```python
from build123d import *

# Parameters (mm, degrees)
F0_W      = 103.65
F0_H      = 64
F0_R      = 1.5
F1_DEPTH  = 1.5
F2_W      = 9
F2_H      = 11
F3_DEPTH  = 16
F4_W      = 7
F4_H      = 7
F4_H_2    = 4
F5_DEPTH  = 1.5
F6_R      = 3.25
F7_DEPTH  = 6
F8_W      = 7
F8_H      = 4.0027049468
F8_H_2    = 1.5
F8_H_3    = 1.4972950532
F9_DEPTH  = 1.5
F10_R     = 3.25
F11_DEPTH = 8
F12_SIZE  = 0.5
F13_SIZE  = 0.5


with BuildPart() as f1:
    # F0 (on Top) → F1 (new body)
    with BuildSketch(Plane.XY):
        Rectangle(F0_W, F0_H)
        with Locations((-48.825, -29)):
            Circle(F0_R, mode=Mode.SUBTRACT)
        with Locations((48.825, -29)):
            Circle(F0_R, mode=Mode.SUBTRACT)
        with Locations((-48.825, 29)):
            Circle(F0_R, mode=Mode.SUBTRACT)
        with Locations((48.825, 29)):
            Circle(F0_R, mode=Mode.SUBTRACT)
    extrude(amount=F1_DEPTH)

    # F2 (on face) → F3 (join)
    with BuildSketch(Plane.YZ.offset(51.825)):
        with Locations((-9.7, 7)):
            Rectangle(F2_W, F2_H)
    extrude(amount=-F3_DEPTH)

    # F4 (on face) → F5 (join)
    with BuildSketch(Plane.YZ.offset(51.825)):
        with Locations((5.9, 2)):
            Rectangle(F4_W, F4_H)
        with Locations((5.9, 3.5)):
            Rectangle(F4_W, F4_H_2)
    extrude(amount=F5_DEPTH)

    # F6 (on face) → F7 (join)
    with BuildSketch(Plane.YZ.offset(53.325)):
        with Locations((5.9, 2)):
            Circle(F6_R)
    extrude(amount=F7_DEPTH)

    # F8 (on face) → F9 (join)
    with BuildSketch(Plane(origin=(-51.825, 0, 0), x_dir=(0, -1, 0), z_dir=(-1, 0, 0))):
        with Locations((-3, 3.5013524734)):
            Rectangle(F8_W, F8_H)
        with Locations((-3, 0.75)):
            Rectangle(F8_W, F8_H_2)
        with Locations((-3, -0.7486475266)):
            Rectangle(F8_W, F8_H_3)
    extrude(amount=F9_DEPTH)

    # F10 (on face) → F11 (join)
    with BuildSketch(Plane(origin=(-53.325, 0, 0), x_dir=(0, -1, 0), z_dir=(-1, 0, 0))):
        with Locations((-3, 2.0027049468)):
            Circle(F10_R)
    extrude(amount=F11_DEPTH)

    # F12
    f12_edges = [f1.edges().sort_by_distance(p)[0] for p in [
        (-61.325, 6.25, 2.002705),
    ]]
    chamfer(f12_edges, length=F12_SIZE)

    # F13
    f13_edges = [f1.edges().sort_by_distance(p)[0] for p in [
        (59.325, 2.65, 2),
    ]]
    chamfer(f13_edges, length=F13_SIZE)


solid = f1.part
```
Can you work these out from the model? Positions are in its coordinate system, mm. A direction names the side the tool comes from. Give positions to 0.01 mm unless a question says otherwise; leave off trailing zeros. Order: outer loops, then holes, each group sorted by start corner. A loop starts at its lowest first (then second) coordinate and runs counter-clockwise, first axis right, second up. Notation, with made-up numbers: (33, -7) - (53, -7) arc R16 cw to (53, 22) - close; hole circle Ø4 at (-27.5, 64). An arc over 180 degrees is marked (long way). Use a Markdown table: item, result. Add a question column.
Q1. Please list where these lines run through material, in increasing order: line 1 along X through (y, z) = (5, 2.75) (3 decimals); line 2 along Z through (x, y) = (25, 24); line 3 along X through (y, z) = (-5.5, 11.25) (3 decimals).
Q2. On a 3-axis mill with a long thin cutter (end or side, diameter ignored), from which of +Z, -Z, +X, -X, +Y, -Y can I reach the whole of each face in a straight line? I mean faces 1 (the cylindrical face through (56.037, 3.321, 0.022)), 2 (the flat face through (44, -5.2, 7)), 3 (the flat face through (51.825, 6, 4)). Say none if no direction works.
Q3. If we section it at A-A on y = -29: Write out the boundary of the cut face in (x, z) (3 decimals).
Q4. I'm going to push flat-ended pins straight in: pin 1 (1.2 mm diameter, centred on x = -52.5, z = 0.5, fed in from -Y); pin 2 (5 mm diameter, centred on x = 48.825, y = 29, fed in from +Z); pin 3 (8 mm diameter, centred on x = 39, y = 12, fed in from -Z). Where does each tip first touch, or does it pass through?
Q5. If we section it at C-C on y = -11.5: Write out the boundary of the cut face in (x, z) (3 decimals), plus the area to 3 significant figures.
Q6. If we section it at D-D on z = 9.5: Write out the boundary of the cut face in (x, y) (3 decimals), plus the area to 3 significant figures.
Q7. If we section it at B-B on x = -49: Write out the boundary of the cut face in (y, z), plus the area to 3 significant figures.
Q8. If we mould it in two halves opening along X, with no side actions, what happens to faces 4 (the flat face through (51.825, -11, 5)), 5 (the cylindrical face through (48.63, -27.513, 0.74)), 6 (the flat face through (-61.325, 3, 2))? For each: released by +X, released by -X, zero draft, split by the parting line, or undercut.
Answers follow:
| question | item | result |
|---|---|---|
| 1 | line 1 | x = -61.325 to -51.825, 51.825 to 59.325 |
| 1 | line 2 | z = 0 to 1.5 |
| 1 | line 3 | x = 35.825 to 51.825 |
| 2 | face 1 | +X |
| 2 | face 2 | +Z, +X, -X, +Y |
| 2 | face 3 | +Z, +Y |
| 3 | outline | (-51.825, 0) - (-50.325, 0) - (-50.325, 1.5) - (-51.825, 1.5) - close; (-47.325, 0) - (47.325, 0) - (47.325, 1.5) - (-47.325, 1.5) - close; (50.325, 0) - (51.825, 0) - (51.825, 1.5) - (50.325, 1.5) - close |
| 4 | pin 1 | stops at y = -0.5 |
| 4 | pin 2 | stops at z = 1.5 |
| 4 | pin 3 | stops at z = 0 |
| 5 | outline | (-51.825, 0) - (51.825, 0) - (51.825, 12.5) - (35.825, 12.5) - (35.825, 1.5) - (-51.825, 1.5) - close |
| 5 | area | 331 mm^2 |
| 6 | outline | (35.825, -14.2) - (51.825, -14.2) - (51.825, -5.2) - (35.825, -5.2) - close |
| 6 | area | 144 mm^2 |
| 7 | outline | (-32, 0) - (-30.49, 0) - (-30.49, 1.5) - (-32, 1.5) - close; (-27.51, 0) - (27.51, 0) - (27.51, 1.5) - (-27.51, 1.5) - close; (30.49, 0) - (32, 0) - (32, 1.5) - (30.49, 1.5) - close |
| 7 | area | 87.1 mm^2 |
| 8 | face 4 | released by +X |
| 8 | face 5 | undercut |
| 8 | face 6 | released by -X |
